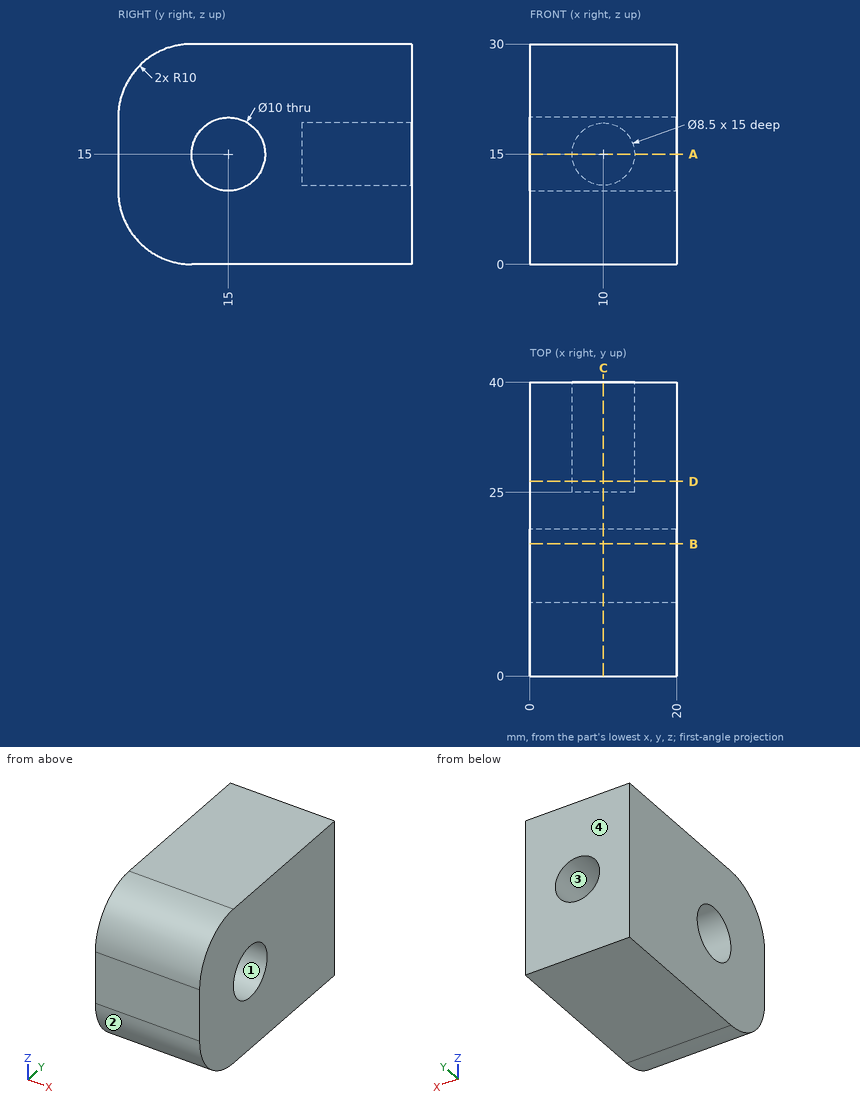
Part print with two shaded views. Sizes in mm from the minimum x, y, z corner. Give positions to 0.01 mm unless a question says otherwise; leave off trailing zeros. Order: outer loops, then holes, each group sorted by start corner. A loop starts at its lowest first (then second) coordinate and runs counter-clockwise, first axis right, second up. Notation, with made-up numbers: (42.25, 49.5) - (56.25, 49.5) arc R38 cw to (56.25, 87.5) - close; hole circle Ø7 at (84.5, 32.25). An arc over 180 degrees is marked (long way). Write each question's results on one line, items separated by ' | '.
1. Saw through at A-A on z = 15. List the corners of the cut face in (x, y).
Calculated:
outline: (0, 0) - (20, 0) - (20, 10) - (0, 10) - close; (0, 20) - (20, 20) - (20, 40) - (14.25, 40) - (14.25, 25) - (5.75, 25) - (5.75, 40) - (0, 40) - close
2. Pull direction Y, two halves, no side cores. Call the marked faces 1, 2, 3 and 4: released by +Y, released by -Y, zero draft, split by the parting line, or undercut.
Calculated:
face 1: undercut | face 2: released by -Y | face 3: zero draft | face 4: released by +Y
3. Saw through at D-D on y = 26.5. List the corners of the cut face in (x, z).
Calculated:
outline: (0, 0) - (20, 0) - (20, 30) - (0, 30) - close; hole circle Ø8.5 at (10, 15)
4. Pin check, flat tips, straight feed: pin 1 (3 mm diameter, centred on x = 6, y = 5, fed in from -Z); pin 2 (3 mm diameter, centred on x = 17, z = 8.5, fed in from -Y). Stop position of each tip, or through.
Calculated:
pin 1: stops at z = 0.63 | pin 2: stops at y = 0
5. Saw through at B-B on y = 18. List the corners of the cut face in (x, z).
Calculated:
outline: (0, 0) - (20, 0) - (20, 11) - (0, 11) - close; (0, 19) - (20, 19) - (20, 30) - (0, 30) - close
6. Probe L1, parallel to X at y = 30, z = 15; L2, parallel to Z at x = 9.75, y = 15; L3, parallel to Y at x = 15.5, z = 15. List the from-to ranges inside material, lowest first. Write a range as from..to.
Calculated:
L1: x = 0..5.75, 14.25..20 | L2: z = 0..10, 20..30 | L3: y = 0..10, 20..40
7. Saw through at C-C on x = 10. List the corners of the cut face in (y, z), and give its area (3 significant figures).
Calculated:
outline: (0, 10) arc R10 ccw to (10, 0) - (40, 0) - (40, 10.75) - (25, 10.75) - (25, 19.25) - (40, 19.25) - (40, 30) - (10, 30) arc R10 ccw to (0, 20) - close; hole circle Ø10 at (15, 15) | area: 951 mm2
